Part model, mm, in its own coordinate system. Face numbers are marked on the shaded views. A direction names the side the tool comes from. Coordinates: 2 decimals unless noted, no trailing zeros. Write each loop counter-clockwise with the first axis right and the second up, starting at its lowest first coordinate (ties: lowest second). Pieces come first, ordered by that corner, then holes. Notation, with made-up numbers: (43, 89) - (95, 89) arc R24 cw to (95, 118) - close; hole circle Ø4 at (-9, 77.25). An arc over 180 degrees is marked (long way). Use a Markdown table: item, result.
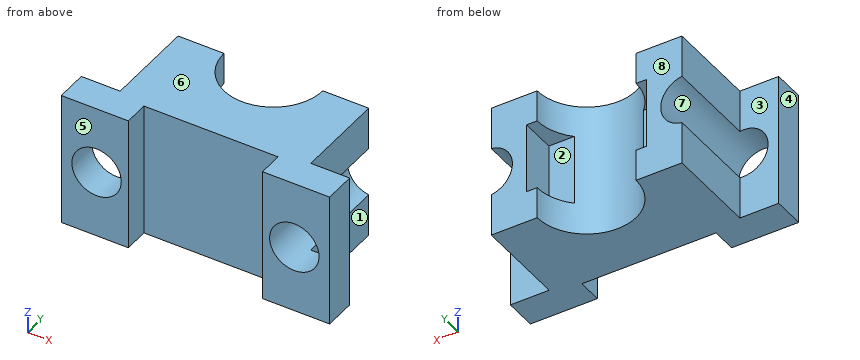
```python
from build123d import *

# Parameters (mm, degrees)
EXTRUDE_1_DEPTH          = 19
CUT_EXTRUDE_1_DEPTH      = 50.809637622
CUT_EXTRUDE_1_DEPTH_BACK = 50.809637622
SKETCH_2_R               = 7
CUT_EXTRUDE_2_DEPTH      = 56.045435778
CUT_EXTRUDE_2_DEPTH_BACK = 10
SKETCH_3_W               = 34
SKETCH_3_H               = 20


with BuildPart() as part:
    # 草图1 → 凸台-拉伸1 (new, symmetric)
    with BuildSketch(Plane.XY):
        with BuildLine():
            ThreePointArc((-14, 35), (0, 21), (14, 35))
            Line((14, 35), (27, 35))
            Line((27, 35), (27, 9))
            Line((27, 9), (38, 9))
            Line((38, 9), (38, 0))
            Line((38, 0), (19, 0))
            Line((19, 0), (19, 7))
            Line((19, 7), (-19, 7))
            Line((-19, 7), (-19, 0))
            Line((-19, 0), (-38, 0))
            Line((-38, 0), (-38, 9))
            Line((-38, 9), (-27, 9))
            Line((-27, 9), (-27, 35))
            Line((-27, 35), (-14, 35))
        make_face()
    extrude(amount=EXTRUDE_1_DEPTH, both=True)

    # 草图2 → 切除-拉伸1 (cut, two sides: drawn at the far end of the back side and taken through both)
    with BuildSketch(Plane(origin=(0, 9, 0), x_dir=(1, 0, 0), z_dir=(0, 1, 0)).offset(-CUT_EXTRUDE_1_DEPTH_BACK)):
        with Locations(Location((28, 0, 0), (0, 0, 270))):
            Circle(SKETCH_2_R)
        with Locations(Location((-28, 0, 0), (0, 0, 278.213210702))):
            Circle(SKETCH_2_R)
    extrude(amount=CUT_EXTRUDE_1_DEPTH + CUT_EXTRUDE_1_DEPTH_BACK, mode=Mode.SUBTRACT)

    # 草图3 → 切除-拉伸2 (cut, two sides: drawn at the far end of the back side and taken through both)
    with BuildSketch(Plane(origin=(0, 35, 0), x_dir=(1, 0, 0), z_dir=(0, 1, 0)).offset(-CUT_EXTRUDE_2_DEPTH_BACK)):
        Rectangle(SKETCH_3_W, SKETCH_3_H)
    extrude(amount=CUT_EXTRUDE_2_DEPTH + CUT_EXTRUDE_2_DEPTH_BACK, mode=Mode.SUBTRACT)


solid = part.part
```
Item 1: Band-saw the part on B-B, the plane z = 0. Give the cut face in (x, y), then the cut area to 3 significant figures.
From the geometry:
| item | result |
|---|---|
| outline | (-38, 0) - (-35, 0) - (-35, 9) - (-38, 9) - close; (-21, 0) - (-19, 0) - (-19, 7) - (19, 7) - (19, 0) - (21, 0) - (21, 35) - (17, 35) - (17, 25) - (9.8, 25) arc R14 cw to (-9.8, 25) - (-17, 25) - (-17, 35) - (-21, 35) - close; (35, 0) - (38, 0) - (38, 9) - (35, 9) - close |
| area | 864 mm^2 |
Item 2: Drop flat-ended pins along their axis: P1, Ø13.5, axis at y = 17, z = 15, coming from the -X side; P2, Ø18, axis at x = -28, z = 0, coming from the -Y side; P3, Ø3.5, axis at x = 12.5, z = 5, coming from the +Y side; P4, Ø8, axis at y = 29.5, z = -1.5, coming from the +X side. Give the stop position or say it passes through.
From the geometry:
| item | result |
|---|---|
| P1 | x = -27 |
| P2 | y = 0 |
| P3 | y = 25 |
| P4 | x = 23.67 |
Item 3: Band-saw the part on D-D, the plane z = -9. Give the cut face in (x, y), then the cut area to 3 significant figures.
From the geometry:
| item | result |
|---|---|
| outline | (-38, 0) - (-19, 0) - (-19, 7) - (19, 7) - (19, 0) - (38, 0) - (38, 9) - (27, 9) - (27, 35) - (17, 35) - (17, 25) - (9.8, 25) arc R14 cw to (-9.8, 25) - (-17, 25) - (-17, 35) - (-27, 35) - (-27, 9) - (-38, 9) - close |
| area | 1,430 mm^2 |
Item 4: Drill centre lines: probe 1 along X at (y, z) = (3.5, 15); probe 2 along X at (y, z) = (27.5, 0); probe 3 along Y at (x, z) = (35, 17). Where is each one in solid material? Low to high.
From the geometry:
| item | result |
|---|---|
| probe 1 | -38 to -19, 19 to 38 |
| probe 2 | -21 to -17, 17 to 21 |
| probe 3 | 0 to 9 |
Item 5: Two-plate mould, pull along Z, no slides. Class the marked faces 6, 7 and 8: pulls with the +Z half, pulls with the -Z half, needs draft (parallel to the pull), parting line crosses it, or undercut.
From the geometry:
| item | result |
|---|---|
| face 6 | pulls with the +Z half |
| face 7 | undercut |
| face 8 | needs draft |
Item 6: Band-saw the part on C-C, the plane y = 19.5. Give the cut face in (x, z), then the cut area to 3 significant figures.
From the geometry:
| item | result |
|---|---|
| outline | (-27, -19) - (27, -19) - (27, -6.93) arc R7 cw to (27, 6.93) - (27, 19) - (-27, 19) - (-27, 6.93) arc R7 cw to (-27, -6.93) - close |
| area | 1,930 mm^2 |
Item 7: Which spindle directions (+Z, -Z, +X, -X, +Y, -Y) get a long thin tool onto all of the face, cutting with end or side? Do the marked faces 1, 2, 3, 4 and 5. Say none if no direction does.
From the geometry:
| item | result |
|---|---|
| face 1 | +Z, -Z, +X, +Y |
| face 2 | +Y |
| face 3 | +Z, -Z, -X, +Y |
| face 4 | +Z, -Z, -X, +Y, -Y |
| face 5 | +Z, -Z, +X, -X, -Y |
Item 8: Band-saw the part on A-A, the plane x = -28. Give the cut face in (y, z), then the cut area to 3 significant figures.
From the geometry:
| item | result |
|---|---|
| outline | (0, -19) - (9, -19) - (9, -7) - (0, -7) - close; (0, 7) - (9, 7) - (9, 19) - (0, 19) - close |
| area | 216 mm^2 |
